```python
from build123d import *

# Parameters (mm, degrees)
F0_W     = 12
F0_H     = 40
F1_DEPTH = 12
F3_DEPTH = 32
F4_DEPTH = 32.001
F5_DEPTH = 32.001
F6_DEPTH = 30.001


with BuildPart() as f1:
    # F0 (on Front) → F1 (new body)
    with BuildSketch(Plane.XZ):
        with BuildLine():
            Line((0, 104.79962), (0, 19.79962))
            ThreePointArc((0, 19.79962), (16, 3.79962), (32, 19.79962))
            Line((32, 19.79962), (32, 104.79962))
            Line((32, 104.79962), (21.593631, 104.79962))
            Line((21.593631, 104.79962), (21.593631, 64.79962))
            Line((21.593631, 64.79962), (9.593631, 64.79962))
            Line((9.593631, 64.79962), (9.593631, 104.79962))
            Line((9.593631, 104.79962), (0, 104.79962))
        make_face()
        with BuildLine():
            Line((9.927311, 19.79962), (9.927311, 44.79962))
            ThreePointArc((9.927311, 44.79962), (15.927311, 50.79962), (21.927311, 44.79962))
            Line((21.927311, 44.79962), (21.927311, 19.79962))
            ThreePointArc((21.927311, 19.79962), (15.927311, 13.79962), (9.927311, 19.79962))
        make_face(mode=Mode.SUBTRACT)
        with Locations((15.593631, 84.79962)):
            Rectangle(F0_W, F0_H)
    extrude(amount=F1_DEPTH)

    # F2 (on face) → F3 (join)
    with BuildSketch(Plane.YZ.offset(32)):
        with BuildLine():
            Line((-12, 94.995772), (-12, 104.496558))
            ThreePointArc((-12, 104.496558), (-29.879182, 91.699606), (-15.789474, 74.82041))
            ThreePointArc((-15.789474, 74.82041), (-13.098095, 73.578943), (-12, 70.825954))
            Line((-12, 70.825954), (-12, 75.102681))
            Line((-12, 75.102681), (-12, 84.603468))
            ThreePointArc((-12, 84.603468), (-21, 89.79962), (-12, 94.995772))
        make_face()
    extrude(amount=-F3_DEPTH)

    # F2 (on face) → F4 (cut, through all)
    with BuildSketch(Plane.YZ.offset(32)):
        with BuildLine():
            ThreePointArc((-9, 89.79962), (-9.803848, 92.79962), (-12, 94.995772))
            Line((-12, 94.995772), (-12, 84.603468))
            ThreePointArc((-12, 84.603468), (-9.803848, 86.79962), (-9, 89.79962))
        make_face()
    extrude(amount=-F4_DEPTH, mode=Mode.SUBTRACT)

    # F2 (on face) → F5 (cut, through all)
    with BuildSketch(Plane.YZ.offset(32)):
        with BuildLine():
            ThreePointArc((-12, 104.496558), (-3.38105, 99.286453), (0, 89.79962))
            Line((0, 89.79962), (0, 104.79962))
            Line((0, 104.79962), (-12, 104.79962))
            Line((-12, 104.79962), (-12, 104.496558))
        make_face()
    extrude(amount=-F5_DEPTH, mode=Mode.SUBTRACT)

    # F0 (on Front) → F6 (cut, through all)
    with BuildSketch(Plane.XZ):
        with Locations((15.593631, 84.79962)):
            Rectangle(F0_W, F0_H)
    extrude(amount=F6_DEPTH, mode=Mode.SUBTRACT)


solid = f1.part
```
Work out the finished part from the listing and answer in its coordinate system (mm). A direction names the side the tool comes from. Round coordinates to 2 decimals unless told otherwise and drop trailing zeros. Write each loop counter-clockwise with the first axis right and the second up, starting at its lowest first coordinate (ties: lowest second). Pieces come first, ordered by that corner, then holes. Notation, with made-up numbers: (-24.5, 81) - (19.5, 81) arc R11 ccw to (19.5, 90) - close; hole circle Ø9 at (81, 55). An arc over 180 degrees is marked (long way). Return JSON: item names as keys, results as strings. Group by question number.
Q1. The part is cut by section A-A on z = 38.5. Write down the section's boundary in (x, y).
Q2. The part is cut by section B-B on x = 16. Write down the section's boundary in (y, z), then the cut area to 3 significant figures.
Q3. Each of these flat-tipped pins is pushed along its axis until it touches: pin 1 Ø6 at (x, y) = (18, -7) entering from +Z; pin 2 Ø2 at (x, y) = (26.5, -17) entering from -Z; pin 3 Ø3 at (x, y) = (6.5, -4) entering from +Z. Where does it stop, or does it pass through?
Q4. The part is cut by section D-D on x = 27. Write down the section's boundary in (y, z).
Q5. The mould has two halves that part along X. Classify faces 1 (the flat face through (21.594, -11, 85)), 2 (the flat face through (0, -11, 72)), 3 (the cylindrical face through (4.86, -13.13, 73.61)), 4 (the flat face through (21.927, -6, 32)): released by +X, released by -X, zero draft, split by the parting line, or undercut.
Q6. Find the intervals of material crossed by L1, parallel to X at y = -6, z = 45; L2, parallel to X at y = -10, z = 72; L3, parallel to Z at x = 28.25, y = -15, in increasing order.
Q7. For faces 5 (the flat face through (9.594, -11, 85)), 6 (the flat face through (32, -11, 71)), 7 (the flat face through (23, -12, 38)), 8 (the cylindrical face through (15.8, -5.9, 50.8)), determine the directions among +Z, -Z, +X, -X, +Y, -Y from which every point of the face is accessible in a straight line to the end or side of a thin tool.
Q8. The part is cut by section C-C on y = -19. Write down the section's boundary in (x, z).
Solved:
{
 "1": {"outline": "(0, -12) - (9.93, -12) - (9.93, 0) - (0, 0) - close; (21.93, -12) - (32, -12) - (32, 0) - (21.93, 0) - close"},
 "2": {"outline": "(-12, 3.8) - (0, 3.8) - (0, 13.8) - (-12, 13.8) - close; (-12, 50.8) - (0, 50.8) - (0, 64.8) - (-12, 64.8) - close", "area": "288 mm²"},
 "3": {"pin 1": "z = 64.8", "pin 2": "z = 74.83", "pin 3": "z = 101.41"},
 "4": {"outline": "(-15.79, 74.82) arc R4 cw to (-12, 70.83) - (-12, 8.18) - (0, 8.18) - (0, 89.8) arc R15 ccw to (-12, 104.5) arc R15 ccw (long way) to start; hole (-12, 84.6) arc R6 ccw to (-9, 89.8) arc R6 ccw to (-12, 95) arc R6 ccw (long way) to start"},
 "5": {"face 1": "undercut", "face 2": "released by -X", "face 3": "zero draft", "face 4": "undercut"},
 "6": {"L1": "0 to 9.93, 21.92 to 32", "L2": "0 to 9.59, 21.59 to 32", "L3": "74.7 to 83.8, 95.8 to 104.8"},
 "7": {"face 5": "+Z, +Y, -Y", "face 6": "+Z, -Z, +X, +Y, -Y", "face 7": "-Z, +X, -X, -Y", "face 8": "+Y, -Y"},
 "8": {"outline": "(0, 75.34) - (9.59, 75.34) - (9.59, 85.33) - (0, 85.33) - close; (0, 94.27) - (9.59, 94.27) - (9.59, 104.26) - (0, 104.26) - close; (21.59, 75.34) - (32, 75.34) - (32, 85.33) - (21.59, 85.33) - close; (21.59, 94.27) - (32, 94.27) - (32, 104.26) - (21.59, 104.26) - close"}
}
